The listing builds one solid part. Answer for the finished solid, in the listing's coordinates (mm). Face numbers are marked on the shaded views. Give positions to 0.01 mm unless a question says otherwise; leave off trailing zeros. Order: outer loops, then holes, each group sorted by start corner. A loop starts at its lowest first (then second) coordinate and runs counter-clockwise, first axis right, second up. Notation, with made-up numbers: M -16.5,-34 L 34.5,-34 A17 ccw 34.5,-9 Z; hole C 46,75.25 d9. An arc over 180 degrees is marked long. Answer as a JSON object with one key per item and string values. Group by question number.
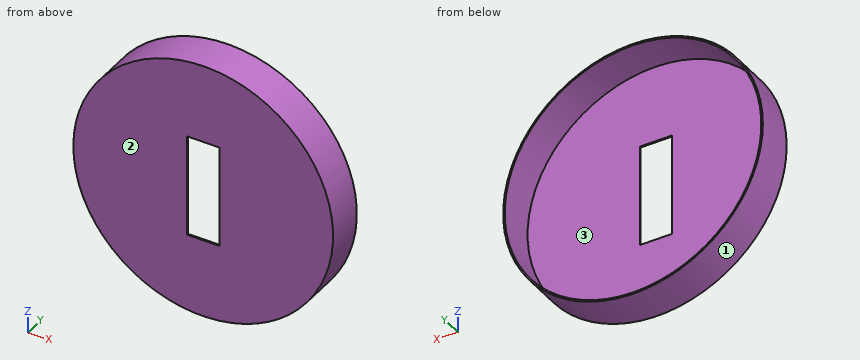
Autodesk Inventor part; units mm, degrees
ref_plane "Work Plane1" through (0, 0, 0) normal (1, 0, 0) x (0, 1, 0)
ref_plane "XZ Plane" through (0, 0, 0) normal (0, 1, 0) x (-1, 0, 0)
ref_plane "XY Plane" through (0, 0, 0) normal (0, 0, 1) x (1, 0, 0)
sketch "Sketch1" plane through (0, 0, 0) normal (0, 1, 0) x (-1, 0, 0)
  circle A0 centre (0, 0) radius 84.5
  line L0 (10.5, 33.25) -> (-10.5, 33.25)
  line L1 (-10.5, 33.25) -> (-10.5, -33.25)
  line L2 (-10.5, -33.25) -> (10.5, -33.25)
  line L3 (10.5, -33.25) -> (10.5, 33.25)
  line L4 (10.5, 33.25) -> (-10.5, -33.25) construction
  line L5 (-10.5, 33.25) -> (10.5, -33.25) construction
  dimension "d0" = 169
  dimension "d1" = 21
  dimension "d2" = 66.5
ref_plane "Work Plane1" through (0, 0, 0) normal (1, 0, 0) x (0, 1, 0)
extrude "Extrusion2" add sketch "Sketch1" along normal blind 25.4
sketch "Sketch3" plane through (0, 25.4, 0) normal (0, 1, 0) x (1, 0, 0)
  circle A0 centre (0, 0) radius 83.5
  dimension "d63" = 167
hole "Hole2" at (0, 25.4, 0) direction (0, -1, 0) diameter 167 depth 24.4
properties part number "Bottom Cap"
Item 1: Section D-D (x = -63.5) is taken. Determine the outline of the cut face in (y, z), and give its area (3 significant figures).
Item 2: Consider probe 1 along Z at (x, y) = (0, 19); probe 2 along X at (y, z) = (16.5, -21). Determine where each line is inside the solid, lowest interval first. Write a range as from..to.
Item 3: Section C-C (y = 21) is taken. Determine the outline of the cut face in (x, z), and give its area (3 significant figures).
Item 4: Flat-ended cylindrical pins translate along their axes: P1, Ø1.5, axis at x = 47.5, z = 58, coming from the -Y side; P2, Ø1.1, axis at x = -2.5, y = 0.5, coming from the +Z side; P3, Ø4, axis at y = 22, z = 23, coming from the -X side; P4, Ø0.8, axis at y = 0.5, z = -6, coming from the +X side. Find the tip coordinate at first contact, or state that the pin passes through.
Item 5: Determine the mould class of the marked faces 1, 2 and 3 for opening direction X: released by +X, released by -X, zero draft, split by the parting line, or undercut.
Item 6: Section B-B (x = 0) is taken. Determine the outline of the cut face in (y, z), and give its area (3 significant figures).
Item 7: Section A-A (z = 0) is taken. Determine the outline of the cut face in (x, y).
Values found:
{
 "1": {"outline": "M 0,-55.75 L 25.4,-55.75 L 25.4,-54.22 L 1,-54.22 L 1,54.22 L 25.4,54.22 L 25.4,55.75 L 0,55.75 Z", "area": "186 mm^2"},
 "2": {"probe 1": "z = -84.5..-83.5, 83.5..84.5", "probe 2": "x = -81.85..-80.82, 80.82..81.85"},
 "3": {"outline": "C 0,0 d169; hole C 0,0 d167", "area": "528 mm^2"},
 "4": {"P1": "stops at y = 0", "P2": "stops at z = 84.48", "P3": "stops at x = -81.85", "P4": "stops at x = 84.31"},
 "5": {"face 1": "split by the parting line", "face 2": "zero draft", "face 3": "undercut"},
 "6": {"outline": "M 0,-84.5 L 25.4,-84.5 L 25.4,-83.5 L 1,-83.5 L 1,-33.25 L 0,-33.25 Z; M 0,33.25 L 1,33.25 L 1,83.5 L 25.4,83.5 L 25.4,84.5 L 0,84.5 Z", "area": "151 mm^2"},
 "7": {"outline": "M -84.5,0 L -10.5,0 L -10.5,1 L -83.5,1 L -83.5,25.4 L -84.5,25.4 Z; M 10.5,0 L 84.5,0 L 84.5,25.4 L 83.5,25.4 L 83.5,1 L 10.5,1 Z"}
}
